```python
from build123d import *

# Parameters (mm, degrees)
F1_DEPTH = 365
F2_R     = 3
F3_R     = 5
F4_W     = 60
F4_H     = 100
F5_DEPTH = 2.7


with BuildPart() as f1:
    # F0 (on Right) → F1 (new body)
    with BuildSketch(Plane.YZ):
        Polygon((0, 0), (0, 2), (-184.4634110061, 2), (0, 108.5), (-1, 110.2320508076), (-191.9275126212, 0), align=None)
    extrude(amount=F1_DEPTH)

    # F2
    f2_edges = [f1.edges().sort_by_distance(p)[0] for p in [
        (182.5, -184.463411, 2),
    ]]
    fillet(f2_edges, radius=F2_R)

    # F3
    f3_edges = [f1.edges().sort_by_distance(p)[0] for p in [
        (182.5, -191.927513, 0),
    ]]
    fillet(f3_edges, radius=F3_R)

    # F4 (on face) → F5 (join)
    with BuildSketch(Plane(origin=(0, -47.9818781553, 83.1070508076), x_dir=(1, 0, 0), z_dir=(0, -0.5, 0.8660254038))):
        with Locations((30, 4.25)):
            Rectangle(F4_W, F4_H)
        with Locations((91, 4.25)):
            Rectangle(F4_W, F4_H)
        with Locations((152, 4.25)):
            Rectangle(F4_W, F4_H)
        with Locations((213, 4.25)):
            Rectangle(F4_W, F4_H)
        with Locations((274, 4.25)):
            Rectangle(F4_W, F4_H)
        with Locations((335, 4.25)):
            Rectangle(F4_W, F4_H)
        with Locations((30, -97.5538475773)):
            Rectangle(F4_W, F4_H)
        with Locations((91, -97.5538475773)):
            Rectangle(F4_W, F4_H)
        with Locations((152, -97.5538475773)):
            Rectangle(F4_W, F4_H)
        with Locations((213, -97.5538475773)):
            Rectangle(F4_W, F4_H)
        with Locations((274, -97.5538475773)):
            Rectangle(F4_W, F4_H)
        with Locations((335, -97.5538475773)):
            Rectangle(F4_W, F4_H)
    extrude(amount=F5_DEPTH)


solid = f1.part
```
Can you work these out from the model? Positions are in its coordinate system, mm. A direction names the side the tool comes from. Coordinates: 2 decimals unless noted, no trailing zeros. Loops run counter-clockwise (first coordinate to the right, second up) from the corner with the lowest first, then second, coordinate; pieces in that order, holes last.
Item 1: I'm going to push flat-ended pins straight in: pin 1 (5 mm diameter, centred on x = 138.5, z = 62.5, fed in from -Y); pin 2 (10 mm diameter, centred on x = 155.5, z = 18, fed in from +Y); pin 3 (3 mm diameter, centred on x = 93.5, y = -151, fed in from +Z). Where does each tip first touch, or does it pass through?
Answers below:
pin 1: stops at y = -93.4
pin 2: stops at y = -148.09
pin 3: stops at z = 27.61
Item 2: Suppose I cut it at A-A (x = 317). Please give me the cut outline in (y, z).
Answers below:
outline: (-177.12, 11.67) - (-175.77, 9.33) arc R5 ccw to (-173.27, 0) - (0, 0) - (0, 2) - (-173.27, 2) arc R3 cw to (-174.77, 7.6) - (0, 108.5) - (-2.35, 112.57) - (-88.95, 62.57) - (-87.6, 60.23) - (-89.16, 59.33) - (-90.51, 61.67) - close
Item 3: Suppose I cut it at C-C (z = 96). Please give me the cut outline in (x, y).
Answers below:
outline: (0, -31.05) - (60, -31.05) - (60, -25.65) - (61, -25.65) - (61, -31.05) - (121, -31.05) - (121, -25.65) - (122, -25.65) - (122, -31.05) - (182, -31.05) - (182, -25.65) - (183, -25.65) - (183, -31.05) - (243, -31.05) - (243, -25.65) - (244, -25.65) - (244, -31.05) - (304, -31.05) - (304, -25.65) - (305, -25.65) - (305, -31.05) - (365, -31.05) - (365, -21.65) - (0, -21.65) - close
Item 4: Which directions (+Z, -Z, +X, -X, +Y, -Y) give clear straight access to the entire face, cutting with the end or side of a thin tool? Please do faces 4 (the face through (122, -134, 35)), 5 (the face through (365, -96, 57)).
Answers below:
face 4: +Z, -Y
face 5: +Z, -Z, +X, +Y, -Y
Item 5: If we mould it in two halves opening along Z, with no side actions, what happens to faces 1 (the face through (334.58, -45.045, 87.92)), 2 (the face through (305, -134, 35)), 3 (the face through (179.94, -88.61, 57.34))? For each: released by +Z, released by -Z, zero draft, split by the parting line, or undercut.
Answers below:
face 1: released by +Z
face 2: zero draft
face 3: undercut
Item 6: Suppose I cut it at B-B (y = -105). Please give me the cut outline in (x, z).
Answers below:
outline: (0, 0) - (365, 0) - (365, 2) - (0, 2) - close; (0, 47.88) - (365, 47.88) - (365, 53.31) - (305, 53.31) - (305, 50.19) - (304, 50.19) - (304, 53.31) - (244, 53.31) - (244, 50.19) - (243, 50.19) - (243, 53.31) - (183, 53.31) - (183, 50.19) - (182, 50.19) - (182, 53.31) - (122, 53.31) - (122, 50.19) - (121, 50.19) - (121, 53.31) - (61, 53.31) - (61, 50.19) - (60, 50.19) - (60, 53.31) - (0, 53.31) - close
Item 7: Please list where these lines run through material, in increasing order: L1, parallel to Z at x = 226, y = -144; L2, parallel to Z at x = 257, y = -81; L3, parallel to Y at x = 252, z = 75.
Answers below:
L1: z = 0 to 2, 25.36 to 30.79
L2: z = 0 to 2, 61.73 to 67.16
L3: y = -67.42 to -58.02
